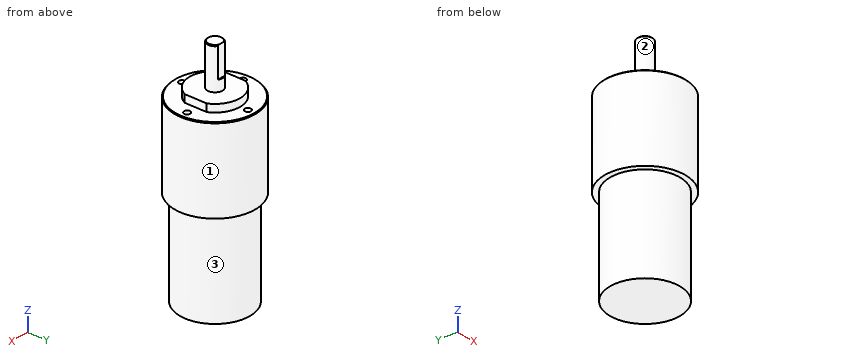
Autodesk Inventor part; units mm, degrees
ref_plane "YZ Plane" through (0, 0, 0) normal (1, 0, 0) x (0, 1, 0)
ref_plane "XZ Plane" through (0, 0, 0) normal (0, 1, 0) x (-1, 0, 0)
ref_plane "XY Plane" through (0, 0, 0) normal (0, 0, 1) x (1, 0, 0)
sketch "スケッチ1" plane through (0, 0, 0) normal (0, 0, 1) x (1, 0, 0)
  circle A0 centre (0, 0) radius 3
  dimension "d0" = 6
extrude "押し出し1" add sketch "スケッチ1" along normal blind 16.3
sketch "スケッチ2" plane through (0, 0, 16.3) normal (0, 0, 1) x (1, 0, 0)
  circle A0 centre (0, 0) radius 3
  line L0 (-1.6583, 2.5) -> (1.6583, 2.5)
  dimension "d3" = 5.5
extrude "押し出し2" cut sketch "スケッチ2" against normal blind 12 contours L0 A0 picked at (-0.1169, 2.6598)
chamfer "面取り1" distance 0.3 angle 45 2 edges at (-1.4186, -2.6434, 16.3) (2.6434, 1.4186, 16.3)
sketch "スケッチ3" plane through (0, 0, 0) normal (0, 0, -1) x (-1, 0, 0)
  circle A0 centre (0, 0) radius 10
  dimension "d9" = 20
extrude "押し出し3" add sketch "スケッチ3" along normal blind 3
sketch "スケッチ4" plane through (0, 0, -3) normal (0, 0, -1) x (-1, 0, 0)
  circle A0 centre (0, 0) radius 10
  line L0 (9, 4.3589) -> (9, -4.3589)
  line L1 (-9, 4.3589) -> (-9, -4.3589)
  dimension "d12" = 18
extrude "押し出し4" cut sketch "スケッチ4" against normal blind 3 contours A0 L0 | L1 A0
sketch "スケッチ5" plane through (0, 0, -3) normal (0, 0, -1) x (-1, 0, 0)
  circle A0 centre (0, 0) radius 16
  dimension "d15" = 32
extrude "押し出し5" add sketch "スケッチ5" along normal blind 33.4
chamfer "面取り2" distance 0.3 angle 45 1 edges at (16, 0, -3)
sketch "スケッチ6" plane through (0, 0, -3) normal (0, 0, 1) x (1, 0, 0)
  arc A0 (9, 4.3589) -> (-9, 4.3589) centre (0, 0) ccw
  point P0 (0, 13)
  point P1 (-13, 0)
  point P2 (0, -13)
  point P3 (13, 0)
  dimension "d21" = 13
  dimension "d24" = 360
hole "穴1" at (0, 13, -3) at (-13, 0, -3) at (0, -13, -3) at (13, 0, -3) direction (0, 0, -1) diameter 2.459 depth 6 tip angle 118
sketch "スケッチ7" plane through (0, 0, -36.4) normal (0, 0, -1) x (-1, 0, 0)
  circle A0 centre (0, 0) radius 13.85
  dimension "d33" = 27.7
extrude "押し出し6" add sketch "スケッチ7" along normal blind 37.8
properties part number "RS385PH_Geared_Motor" material "鋼、鍛鋼"
Model file for the job. Use its own axes, mm. Face numbers are marked on the shaded views. A direction names the side the tool comes from. Coordinates: 2 decimals unless noted, no trailing zeros. Write each loop counter-clockwise with the first axis right and the second up, starting at its lowest first coordinate (ties: lowest second). Pieces come first, ordered by that corner, then holes. Notation, with made-up numbers: (54, 72.25) - (76, 72.25) arc R20 ccw to (76, 111.25) - close; hole circle Ø6 at (-39, 5.25). An arc over 180 degrees is marked (long way). One line per item, written item: value. Start each with the question number.
1. Slice it at C-C (z = -27). Write the cut outline in (x, y), plus the area to 3 significant figures.
2. Slice it at B-B (z = -64.5). Write the cut outline in (x, y), plus the area to 3 significant figures.
3. Slice it at A-A (z = 7.5). Write the cut outline in (x, y).
4. Flat gauge pins, fed straight in: pin 1 (6 mm diameter, centred on x = -9.5, z = -62, fed in from -Y); pin 2 (2 mm diameter, centred on x = -10.5, z = -49.5, fed in from +Y); pin 3 (5 mm diameter, centred on y = -6.5, z = -6, fed in from +X). Where does each tip first touch, or does it go through?
5. Tool access for the marked faces 1, 2 and 3: list every direction of +Z, -Z, +X, -X, +Y, -Y with a clear straight run to the whole face (end or side of a thin tool).
6. Probe line 1 (Y direction, x = 0, z = -5.9); line 2 (Z direction, x = 6.5, y = -11); line 3 (Z direction, x = -5, y = 7.5). List the from-to ranges inside material, lowest first. Write a range as from..to.
Answers below:
1. outline: circle Ø32 at (0, 0)
1. area: 804 mm^2
2. outline: circle Ø27.7 at (0, 0)
2. area: 603 mm^2
3. outline: (-1.66, 2.5) arc R3 ccw (long way) to (1.66, 2.5) - close
4. pin 1: stops at y = -12.23
4. pin 2: stops at y = 10.08
4. pin 3: stops at x = 15.49
5. face 1: +Z, -Z
5. face 2: +Z
5. face 3: -Z
6. line 1: y = -16..-14.23, -11.77..11.77, 14.23..16
6. line 2: z = -74.2..-3
6. line 3: z = -74.2..0
